Can you work these out from the model? Positions are in its coordinate system, mm. Face numbers are marked on the shaded views. A direction names the side the tool comes from. Give positions to 0.01 mm unless a question says otherwise; leave off trailing zeros. Loops run counter-clockwise (first coordinate to the right, second up) from the corner with the lowest first, then second, coordinate; pieces in that order, holes last. Notation, with made-up numbers: M 0.25,41 L 32.25,41 A14 ccw 32.25,46 Z; hole C 77.25,88.5 d11. An arc over 180 degrees is marked long. Use CSV: the item, a comma, the result in double quotes.
from build123d import *

# Parameters (mm, degrees)
F0_W     = 156.0007420911
F0_H     = 75.5530648724
F1_DEPTH = 25
F2_W     = 46.8510948122
F2_H     = 75.7792815566
F3_DEPTH = 1
F5_D     = 20
F7_DEPTH = 255
F8_W     = 83.6402047426
F8_H     = 32.7123841271
F9_DEPTH = 100


with BuildPart() as f1:
    # F0 (on Top) → F1 (new body)
    with BuildSketch(Plane.XY):
        with BuildLine():
            Line((84.4286978245, 53.1719140444), (-77.1694108844, 53.1719140444))
            ThreePointArc((-77.1694108844, 53.1719140444), (-89.2789735535, 46.929714102), (-94.6344383061, 34.4027206302))
            Line((-94.6344383061, 34.4027206302), (-94.6344383061, -28.4059178084))
            ThreePointArc((-94.6344383061, -28.4059178084), (-81.8076298673, -56.6572698383), (-58.2321323454, -76.8280859556))
            Line((-58.2321323454, -76.8280859556), (-13.4139051661, -76.8280859556))
            ThreePointArc((-13.4139051661, -76.8280859556), (-11.9224470417, -69.5865469722), (-8.3639649674, -63.105687499))
            Line((-8.3639649674, -63.105687499), (12.4670406803, -63.105687499))
            ThreePointArc((12.4670406803, -63.105687499), (17.0740541232, -69.2355741117), (18.1482266635, -76.8280859556))
            Line((18.1482266635, -76.8280859556), (71.4882239699, -76.8280859556))
            ThreePointArc((71.4882239699, -76.8280859556), (95.5316118327, -57.587637734), (105.3655616939, -28.4059178084))
            Line((105.3655616939, -28.4059178084), (105.3655616939, 35.0339636207))
            ThreePointArc((105.3655616939, 35.0339636207), (99.0954169594, 47.7024097941), (86.0612784494, 53.1719140444))
            Line((86.0612784494, 53.1719140444), (84.4286978245, 53.1719140444))
        make_face()
        with Locations((3.4495101505, -4.5515570394)):
            Rectangle(F0_W, F0_H, mode=Mode.SUBTRACT)
    extrude(amount=F1_DEPTH)

    # F2 (on Top) → F3 (join)
    with BuildSketch(Plane.XY):
        with Locations((-0.2943016589, -4.5300647616)):
            Rectangle(F2_W, F2_H)
    extrude(amount=F3_DEPTH)

    # F5 (through all)
    with Locations(Plane(origin=(0, 0, 0), x_dir=(1, 0, 0), z_dir=(0, 0, -1))):
        with Locations((0, 0)):
            Hole(F5_D / 2)

    # F6 (on face) → F7 (cut)
    with BuildSketch(Plane(origin=(0, 53.1719140444, 0), x_dir=(-1, 0, 0), z_dir=(0, 1, 0))):
        with BuildLine():
            Line((20.4541144112, 28.5491645336), (0, 25))
            add(Edge.make_bspline(
                [(0, 25), (26.840212886, 25.1204533791), (71.8387888182, 24.3904514867), (100.6753190799, 18.4198146688), (107.8883484006, 15.5325448141)],
                knots=[0, 0, 0, 0, 0.5988321729, 1, 1, 1, 1], degree=3))
            Line((107.8883484006, 15.5325448141), (107.8883484006, 28.5491645336))
            Line((107.8883484006, 28.5491645336), (20.4541144112, 28.5491645336))
        make_face()
        with BuildLine():
            add(Edge.make_bspline(
                [(0, 25), (-26.840212886, 25.1204533791), (-71.8387888182, 24.3904514867), (-100.6753190799, 18.4198146688), (-107.8883484006, 15.5325448141)],
                knots=[0, 0, 0, 0, 0.5988321729, 1, 1, 1, 1], degree=3))
            Line((0, 25), (-20.4541144112, 28.5491645336))
            Line((-20.4541144112, 28.5491645336), (-107.8883484006, 28.5491645336))
            Line((-107.8883484006, 28.5491645336), (-107.8883484006, 15.5325448141))
        make_face()
    extrude(amount=-F7_DEPTH, mode=Mode.SUBTRACT)

    # F8 (on Front) → F9 (cut, symmetric)
    with BuildSketch(Plane.XZ):
        with Locations((-66.6241189465, 2.2455067374)):
            Rectangle(F8_W, F8_H)
        with Locations((66.6241189465, 2.2455067374)):
            Rectangle(F8_W, F8_H)
    extrude(amount=F9_DEPTH, both=True, mode=Mode.SUBTRACT)


solid = f1.part
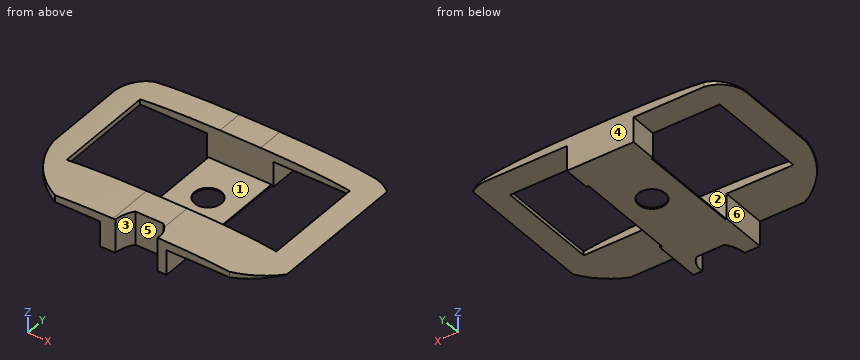
Q1. I'm going to push flat-ended pins straight in: P1, Ø4, axis at y = -40.5, z = 12.5, coming from the +X side; P2, Ø0.5, axis at y = -3, z = 0.5, coming from the -X side; P3, Ø1, axis at x = -44.5, y = -60, coming from the -Z side. Where does each tip first touch, or does it pass through?
Model answer:
P1,"x = 24.8"
P2,"x = -23.72"
P3,"z = 18.6"
Q2. For the marked faces 1, 2 and 3, which set-ups out of +Z, -Z, +X, -X, +Y, -Y let a thin tool reach every point of the face, with its end or its side?
Model answer:
face 1,"+Z, +X, -X"
face 2,"+Z"
face 3,"+Z, -Z, -Y"
Q3. Please list where these lines run through material, in increasing order: L1, parallel to Y at x = 0, z = 0.3; L2, parallel to Z at x = -10.5, y = -27.5; L3, parallel to X at y = -55, z = 4. Write a range as from..to.
Model answer:
L1,"-63.11..-10, 10..53.17"
L2,"0..1"
L3,"-24.8..24.8"
Q4. I want a section at C-C, the plane y = 0. State how many separate pieces and enclosed holes the cut face has, then the cut area to 3 significant figures.
Model answer:
separate pieces,"4"
enclosed holes,"0"
area,"102 mm2"
Q5. If we mould it in two halves opening along X, with no side actions, what happens to the marked faces 4, 5 and 6? For each: released by +X, released by -X, zero draft, split by the parting line, or undercut.
Model answer:
face 4,"zero draft"
face 5,"undercut"
face 6,"released by -X"
Q6. I want a section at B-B, the plane x = 0. Please give me the cut outline in (y, z).
Model answer:
outline,"M -63.11,0 L -10,0 L -10,1 L -42.33,1 L -42.33,25 L -63.11,25 Z; M 10,0 L 53.17,0 L 53.17,25 L 33.22,25 L 33.22,1 L 10,1 Z"
Q7. I want a section at A-A, the plane z = 6.5. Please give me the cut outline in (x, y), then the cut area to 3 significant figures.
Model answer:
outline,"M -24.8,-76.83 L -13.41,-76.83 A24.82 cw -8.36,-63.11 L 12.47,-63.11 A15.38 cw 18.15,-76.83 L 24.8,-76.83 L 24.8,-42.33 L -24.8,-42.33 Z; M -24.8,33.22 L 24.8,33.22 L 24.8,53.17 L -24.8,53.17 Z"
area,"2,310 mm2"
